Check sheet for the modelled part. Datum: model origin and axes. Units: mm. Face numbers are marked on the shaded views. Round coordinates to 2 decimals unless told otherwise and drop trailing zeros. Loops run counter-clockwise (first coordinate to the right, second up) from the corner with the lowest first, then second, coordinate; pieces in that order, holes last. Notation, with made-up numbers: (60.5, 35) -> (91.5, 35) arc R27 cw to (91.5, 62) -> close; hole circle Ø10 at (30, -34.5). An arc over 180 degrees is marked (long way). Use one line per item in the form item = value. Start each with the question number.
(1) Go/stop test with flat-tipped pins: pin 1 (5 mm diameter, centred on x = 3, z = 197, fed in from +Y); pin 2 (6 mm diameter, centred on x = 11.5, z = 73.5, fed in from +Y); pin 3 (3.5 mm diameter, centred on x = 5, y = 153, fed in from +Z); pin 4 (3.5 mm diameter, centred on x = 7, y = 194, fed in from -Z). Record where each tip stops, or that it passes through.
(2) Sectioned sample at A-A (y = 33). State how many separate pieces and enclosed holes the cut face has, and give its area (3 significant figures).
(3) Draft check along Z on the marked faces 1 and 2. Enter one of: released by +Z, released by -Z, zero draft, split by the parting line, or undercut.
(4) Sectioned sample at C-C (y = 106). Record the cut outline in (x, z), and give its area (3 significant figures).
(5) Sectioned sample at B-B (z = 51). Record the cut outline in (x, y).
(6) Material ranges on probe 1 along Y at (x, z) = (5, 209.45); probe 2 along Z at (x, y) = (7, 22.5); probe 3 along X at (y, z) = (153, 0.55), recorded low to high. Write a range as [from, to].
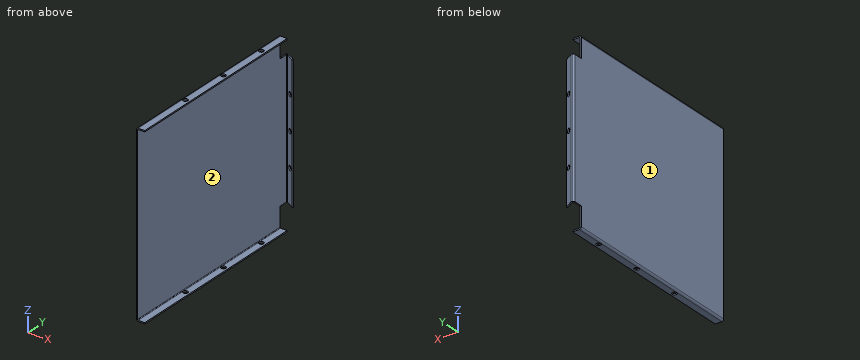
from build123d import *

# Parameters (mm, degrees)
SKETCH_1_W                       = 1.5
SKETCH_1_H                       = 200
SM_BASE_FLANGE_1_DEPTH           = 210
SM_EDGE_FLANGE_2_DEPTH           = 210
SM_EDGE_FLANGE_2_2_DEPTH         = 210
CUT_EXTRUDE_1_DEPTH              = 25
SKETCH_13_W                      = 1.5
SKETCH_13_H                      = 25
CUT_EXTRUDE_2_DEPTH              = 10
SKETCH_14_R                      = 2.75
CUT_EXTRUDE_3_DEPTH              = 10
SM_EDGE_FLANGE_5_STRIP_W         = 7.4732
SM_EDGE_FLANGE_5_STRIP_H         = 1.5
SM_EDGE_FLANGE_5_STRIP_CUT_DEPTH = 186.992120568
SM_EDGE_FLANGE_5_DEPTH           = 186.992120568
SM_EDGE_FLANGE_6_STRIP_W         = 7.4732
SM_EDGE_FLANGE_6_STRIP_H         = 1.5
SM_EDGE_FLANGE_6_STRIP_CUT_DEPTH = 186.992120568
SM_EDGE_FLANGE_6_DEPTH           = 186.992120568
SKETCH_27_R                      = 2.75
CUT_EXTRUDE_4_DEPTH              = 290.759957722
EXTRUDE_1_DEPTH                  = 38


# Read off the part's stored shape, not the designer's step: 边线-法兰2
# Sheet-metal steps are written as plain solids
with BuildPart() as part:
    # Sketch 1 → 基体-法兰1 (new body)
    with BuildSketch(Plane.XY):
        with Locations((0.75, 100)):
            Rectangle(SKETCH_1_W, SKETCH_1_H)
    extrude(amount=SM_BASE_FLANGE_1_DEPTH)

    # 边线-法兰2 outline → 边线-法兰2 (cut)
    with BuildSketch(Plane.XY):
        with BuildLine():
            ThreePointArc((0, 196.992120568), (0.413161062, 198.28728465), (1.5, 199.103944424))
            Line((1.5, 199.103944424), (1.5, 200))
            Line((1.5, 200), (0, 200))
            Line((0, 200), (0, 196.992120568))
        make_face()
    extrude(amount=SM_EDGE_FLANGE_2_DEPTH, mode=Mode.SUBTRACT)

    # Sm Edge Flange 2 2 outline → Sm Edge Flange 2 2 (add)
    with BuildSketch(Plane.XY):
        with BuildLine():
            Line((12.990381057, 193.366025404), (3.3549, 198.929072986))
            ThreePointArc((3.3549, 198.929072986), (2.446525528, 199.218847051), (1.5, 199.103944424))
            Line((1.5, 199.103944424), (1.5, 196.992120568))
            ThreePointArc((1.5, 196.992120568), (1.8683, 197.63003488), (2.6049, 197.63003488))
            Line((2.6049, 197.63003488), (12.240381057, 192.066987298))
            Line((12.240381057, 192.066987298), (12.990381057, 193.366025404))
        make_face()
    extrude(amount=SM_EDGE_FLANGE_2_2_DEPTH)

    # 草图12 → 切除-拉伸1 (cut)
    with BuildSketch(Plane(origin=(0, 0, 0), x_dir=(-1, 0, 0), z_dir=(0, 0, -1))):
        Polygon((0, 196.992120568), (-3.169381215, 196.992120568), (-3.169381215, 190.456162681), (-17.36722667, 190.456162681), (-17.36722667, 200.115352772), (-3.169381215, 200.115352772), (0, 200.115352772), align=None)
    cut_extrude_1 = extrude(amount=-CUT_EXTRUDE_1_DEPTH, mode=Mode.SUBTRACT)

    # 草图13 → 切除-拉伸2 (cut)
    with BuildSketch(Plane(origin=(0, 196.992120568, 0), x_dir=(1, 0, 0), z_dir=(0, 1, 0))):
        with Locations((0.75, -12.5)):
            Rectangle(SKETCH_13_W, SKETCH_13_H)
    cut_extrude_2 = extrude(amount=-CUT_EXTRUDE_2_DEPTH, mode=Mode.SUBTRACT)

    # 镜向1: 切除-拉伸1, 切除-拉伸2 across plane
    add(cut_extrude_1.mirror(Plane(origin=(0, 0, 105), x_dir=(1, 0, 0), z_dir=(0, 0, -1))), mode=Mode.SUBTRACT)
    add(cut_extrude_2.mirror(Plane(origin=(0, 0, 105), x_dir=(1, 0, 0), z_dir=(0, 0, -1))), mode=Mode.SUBTRACT)

    # 草图14 → 切除-拉伸3 (cut)
    with BuildSketch(Plane(origin=(86.227540378, 149.350480947, 0), x_dir=(0.86602540378444, -0.4999999999999978, 0), z_dir=(-0.4999999999999978, -0.86602540378444, 0))):
        with Locations((-90.996060284, 65)):
            Circle(SKETCH_14_R)
        with Locations((-90.996060284, 105)):
            Circle(SKETCH_14_R)
        with Locations(Location((-90.996060284, 145, 0), (0, 0, 180))):
            Circle(SKETCH_14_R)
    extrude(amount=-CUT_EXTRUDE_3_DEPTH, mode=Mode.SUBTRACT)

    # 边线-法兰5 strip (across the edge) → 边线-法兰5 strip cut (cut)
    with BuildSketch(Plane(origin=(1.5, 0, 0), x_dir=(0, 0, 1), z_dir=(0, 1, 0))):
        with Locations((-1.5, -0.75)):
            Rectangle(SM_EDGE_FLANGE_5_STRIP_W, SM_EDGE_FLANGE_5_STRIP_H)
    extrude(amount=SM_EDGE_FLANGE_5_STRIP_CUT_DEPTH, mode=Mode.SUBTRACT)

    # 边线-法兰5 section (across the edge) → 边线-法兰5 (add)
    with BuildSketch(Plane(origin=(1.5, 0, 0), x_dir=(0, 0, 1), z_dir=(0, 1, 0))):
        with BuildLine():
            Line((0, 0.7366), (0, 8.5))
            Line((0, 8.5), (1.5, 8.5))
            Line((1.5, 8.5), (1.5, 0.7366))
            ThreePointArc((1.5, 0.7366), (1.715745145, 0.215745145), (2.2366, 0))
            Line((2.2366, 0), (2.2366, -1.5))
            ThreePointArc((2.2366, -1.5), (0.655084973, -0.844915027), (0, 0.7366))
        make_face()
    extrude(amount=SM_EDGE_FLANGE_5_DEPTH)

    # 边线-法兰6 strip (across the edge) → 边线-法兰6 strip cut (cut)
    with BuildSketch(Plane(origin=(1.5, 186.992120568, 210), x_dir=(0, 0, -1), z_dir=(0, -1, 0))):
        with Locations((-1.5, -0.75)):
            Rectangle(SM_EDGE_FLANGE_6_STRIP_W, SM_EDGE_FLANGE_6_STRIP_H)
    extrude(amount=SM_EDGE_FLANGE_6_STRIP_CUT_DEPTH, mode=Mode.SUBTRACT)

    # 边线-法兰6 section (across the edge) → 边线-法兰6 (add)
    with BuildSketch(Plane(origin=(1.5, 186.992120568, 210), x_dir=(0, 0, -1), z_dir=(0, -1, 0))):
        with BuildLine():
            Line((0, 0.7366), (0, 8.5))
            Line((0, 8.5), (1.5, 8.5))
            Line((1.5, 8.5), (1.5, 0.7366))
            ThreePointArc((1.5, 0.7366), (1.715745145, 0.215745145), (2.2366, 0))
            Line((2.2366, 0), (2.2366, -1.5))
            ThreePointArc((2.2366, -1.5), (0.655084973, -0.844915027), (0, 0.7366))
        make_face()
    extrude(amount=SM_EDGE_FLANGE_6_DEPTH)

    # 草图27 → 切除-拉伸4 (cut, through all)
    with BuildSketch(Plane(origin=(0, 0, 0), x_dir=(-1, 0, 0), z_dir=(0, 0, -1))):
        with Locations((-5, 153)):
            Circle(SKETCH_27_R)
        with Locations((-5, 93)):
            Circle(SKETCH_27_R)
        with Locations((-5, 33)):
            Circle(SKETCH_27_R)
    extrude(amount=-CUT_EXTRUDE_4_DEPTH, mode=Mode.SUBTRACT)

    # 草图28 → 凸台-拉伸1 (add)
    with BuildSketch(Plane.XZ):
        with BuildLine():
            Line((0, 2.2366), (0, 207.7634))
            ThreePointArc((0, 207.7634), (0.655084973, 209.344915027), (2.2366, 210))
            Line((2.2366, 210), (10, 210))
            Line((10, 210), (10, 208.5))
            Line((10, 208.5), (2.2366, 208.5))
            ThreePointArc((2.2366, 208.5), (1.715745145, 208.284254855), (1.5, 207.7634))
            Line((1.5, 207.7634), (1.5, 2.2366))
            ThreePointArc((1.5, 2.2366), (1.715745145, 1.715745145), (2.2366, 1.5))
            Line((2.2366, 1.5), (10, 1.5))
            Line((10, 1.5), (10, 0))
            Line((10, 0), (2.2366, 0))
            ThreePointArc((2.2366, 0), (0.655084973, 0.655084973), (0, 2.2366))
        make_face()
    extrude(amount=EXTRUDE_1_DEPTH)


solid = part.part
Checks:
q1.pin_1 = 186.99
q1.pin_2 = 195.96
q1.pin_3 = through
q1.pin_4 = 25
q2.separate_pieces = 3
q2.enclosed_holes = 0
q2.area = 322 mm2
q3.face_1 = zero draft
q3.face_2 = undercut
q4.outline = (0, 2.24) arc R2.24 ccw to (2.24, 0) -> (10, 0) -> (10, 1.5) -> (2.24, 1.5) arc R0.74 cw to (1.5, 2.24) -> (1.5, 207.76) arc R0.74 cw to (2.24, 208.5) -> (10, 208.5) -> (10, 210) -> (2.24, 210) arc R2.24 ccw to (0, 207.76) -> close
q4.area = 339 mm2
q5.outline = (0, -38) -> (1.5, -38) -> (1.5, 196.99) arc R0.74 cw to (2.6, 197.63) -> (12.24, 192.07) -> (12.99, 193.37) -> (3.35, 198.93) arc R2.24 ccw to (0, 196.99) -> close
q6.probe_1 = [-38, 30.25], [35.75, 90.25], [95.75, 150.25], [155.75, 186.99]
q6.probe_2 = [0, 1.5], [208.5, 210]
q6.probe_3 = [0.77, 2.25], [7.75, 10]
